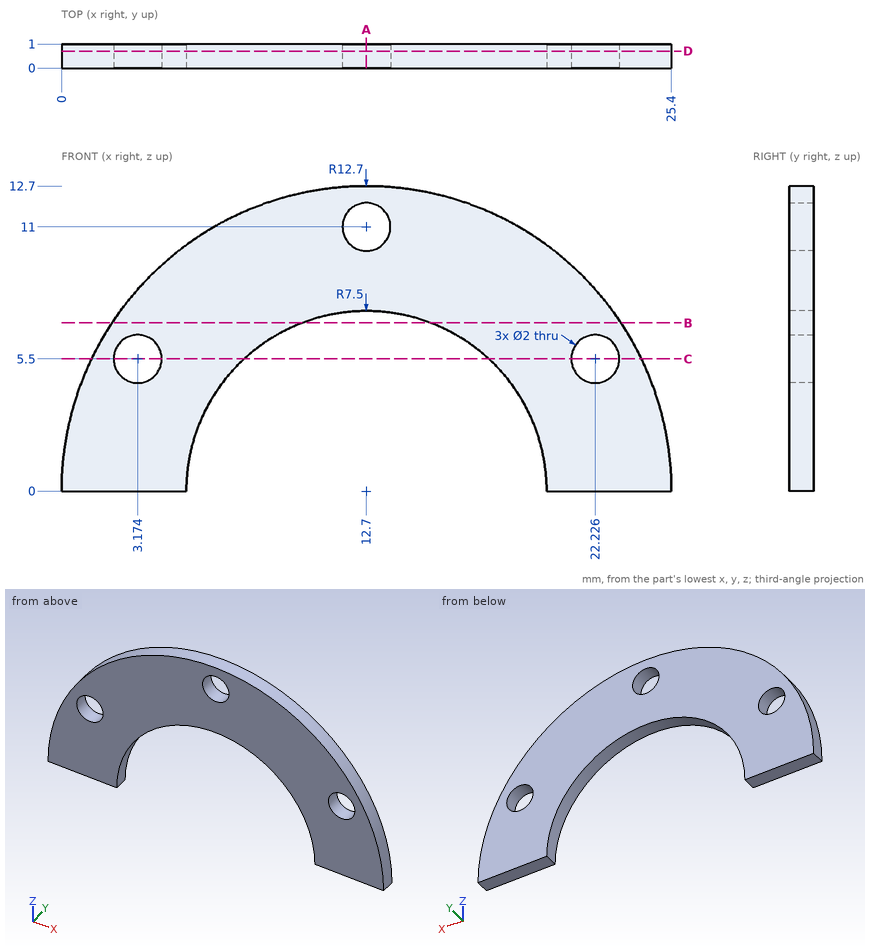
Check sheet for the drawn part. Datum: minimum x, y, z corner. Units: mm. Give positions to 0.01 mm unless a question says otherwise; leave off trailing zeros. Write each loop counter-clockwise with the first axis right and the second up, starting at its lowest first coordinate (ties: lowest second). Pieces come first, ordered by that corner, then holes. Notation, with made-up numbers: M -16,46.5 L 9,46.5 A18 cw 9,60.5 Z; hole C 57.5,62 d6. An arc over 180 degrees is marked long. One line per question, with ' | ' between items.
1. Cross-section at C-C (z = 5.5). Enter the section's corners in (x, y).
Ans:
outline: M 1.25,0 L 2.17,0 L 2.17,1 L 1.25,1 Z; M 4.17,0 L 7.6,0 L 7.6,1 L 4.17,1 Z; M 17.8,0 L 21.23,0 L 21.23,1 L 17.8,1 Z; M 23.23,0 L 24.15,0 L 24.15,1 L 23.23,1 Z
2. Cross-section at A-A (x = 12.7). Enter the section's corners in (y, z).
Ans:
outline: M 0,7.5 L 1,7.5 L 1,10 L 0,10 Z; M 0,12 L 1,12 L 1,12.7 L 0,12.7 Z
3. Cross-section at D-D (y = 0.7). Enter the section's corners in (x, z), plus the area to 3 significant figures.
Ans:
outline: M 0,0 L 5.2,0 A7.5 cw 20.2,0 L 25.4,0 A12.7 ccw Z; hole C 3.17,5.5 d2; hole C 12.7,11 d2; hole C 22.23,5.5 d2 | area: 156 mm2
4. Cross-section at B-B (z = 7). Enter the section's corners in (x, y).
Ans:
outline: M 2.1,0 L 10.01,0 L 10.01,1 L 2.1,1 Z; M 15.39,0 L 23.3,0 L 23.3,1 L 15.39,1 Z
5. Scan lines: line 1 along X through (y, z) = (0.85, 5.5) (1 decimal); line 2 along Z through (x, y) = (12.7, 0.4); line 3 along Z through (x, y) = (23, 0.7) (1 decimal). Record each from-to range of solid material in increasing order. Write a range as from..to.
Ans:
line 1: 1.3..2.2, 4.2..7.6, 17.8..21.2, 23.2..24.1 | line 2: 7.5..10, 12..12.7 | line 3: 0..4.9, 6.1..7.4
